Geometry: final body of the model. Coordinates: model frame, mm. Face numbers are marked on the shaded views. A direction names the side the tool comes from. Give positions to 0.01 mm unless a question says otherwise; leave off trailing zeros. Loops run counter-clockwise (first coordinate to the right, second up) from the corner with the lowest first, then second, coordinate; pieces in that order, holes last. Notation, with made-up numbers: (39, 81.25) - (47, 81.25) arc R27 cw to (47, 105.25) - close; hole circle Ø3 at (-3, 83.5). An arc over 180 degrees is marked (long way). Use one line per item in the form item = value.
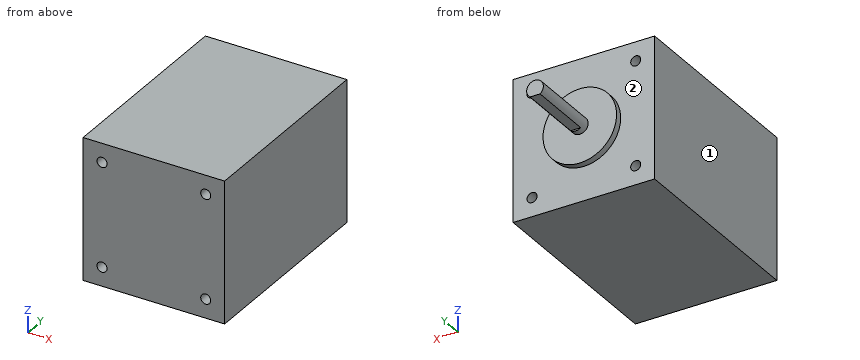
```python
from build123d import *

# Parameters (mm, degrees)
SKETCH_1_W          = 42.3
SKETCH_1_H          = 42.3
SKETCH_1_R          = 1.5
EXTRUDE_1_DEPTH     = 60
SKETCH_2_R          = 11
EXTRUDE_2_DEPTH     = 2
SKETCH_3_R          = 2.5
EXTRUDE_3_DEPTH     = 22
SKETCH_4_W          = 5
SKETCH_4_H          = 0.5
CUT_EXTRUDE_1_DEPTH = 20


with BuildPart() as part:
    # Эскиз1 → Бобышка-Вытянуть1 (new body)
    with BuildSketch(Plane(origin=(0, 0, 0), x_dir=(1, 0, 0), z_dir=(0, 1, 0))):
        with Locations((21.15, 21.15)):
            Rectangle(SKETCH_1_W, SKETCH_1_H)
        with Locations(Location((5.65, 36.65, 0), (0, 0, 270))):
            Circle(SKETCH_1_R, mode=Mode.SUBTRACT)
        with Locations(Location((36.65, 36.65, 0), (0, 0, 270))):
            Circle(SKETCH_1_R, mode=Mode.SUBTRACT)
        with Locations(Location((36.65, 5.65, 0), (0, 0, 270))):
            Circle(SKETCH_1_R, mode=Mode.SUBTRACT)
        with Locations(Location((5.65, 5.65, 0), (0, 0, 270))):
            Circle(SKETCH_1_R, mode=Mode.SUBTRACT)
    extrude(amount=EXTRUDE_1_DEPTH)

    # Эскиз2 → Бобышка-Вытянуть2 (add)
    with BuildSketch(Plane(origin=(0, 60, 0), x_dir=(1, 0, 0), z_dir=(0, 1, 0))):
        with Locations(Location((21.15, 21.15, 0), (0, 0, 90))):
            Circle(SKETCH_2_R)
    extrude(amount=EXTRUDE_2_DEPTH)

    # Эскиз3 → Бобышка-Вытянуть3 (add)
    with BuildSketch(Plane(origin=(0, 62, 0), x_dir=(1, 0, 0), z_dir=(0, 1, 0))):
        with Locations(Location((21.15, 21.15, 0), (0, 0, 270))):
            Circle(SKETCH_3_R)
    extrude(amount=EXTRUDE_3_DEPTH)

    # Эскиз4 → Вырез-Вытянуть1 (cut)
    with BuildSketch(Plane(origin=(0, 84, 0), x_dir=(1, 0, 0), z_dir=(0, 1, 0))):
        with Locations((21.15, 23.4)):
            Rectangle(SKETCH_4_W, SKETCH_4_H)
    extrude(amount=-CUT_EXTRUDE_1_DEPTH, mode=Mode.SUBTRACT)


solid = part.part
```
(1) Material intervals for L1, parallel to X at y = 23, z = -5.65; L2, parallel to X at y = 18, z = -36; L3, parallel to Z at x = 5, y = 31, sorted ascending. Write a range as from..to.
Solution:
L1 = 0..4.15, 7.15..35.15, 38.15..42.3
L2 = 0..4.3, 7..35.3, 38..42.3
L3 = -42.3..-38, -35.3..-7, -4.3..0
(2) Cut plane A-A (y = 28). Return the cut outline in (x, z).
Solution:
outline = (0, -42.3) - (42.3, -42.3) - (42.3, 0) - (0, 0) - close; hole circle Ø3 at (5.65, -36.65); hole circle Ø3 at (5.65, -5.65); hole circle Ø3 at (36.65, -36.65); hole circle Ø3 at (36.65, -5.65)
(3) Cut plane B-B (x = 5.65). Return the cut outline in (y, z), plus the area to 3 significant figures.
Solution:
outline = (0, -42.3) - (60, -42.3) - (60, -38.15) - (0, -38.15) - close; (0, -35.15) - (60, -35.15) - (60, -7.15) - (0, -7.15) - close; (0, -4.15) - (60, -4.15) - (60, 0) - (0, 0) - close
area = 2,180 mm2
(4) Cut plane C-C (z = -5.65). Return the cut outline in (x, y), plus the area to 3 significant figures.
Solution:
outline = (0, 0) - (4.15, 0) - (4.15, 60) - (0, 60) - close; (7.15, 0) - (35.15, 0) - (35.15, 60) - (7.15, 60) - close; (38.15, 0) - (42.3, 0) - (42.3, 60) - (38.15, 60) - close
area = 2,180 mm2
(5) Pin query (flat end, axial travel): P1, Ø2.5, axis at x = 5.65, z = -5.65, coming from the -Y side; P2, Ø12, axis at x = 33, z = -34, coming from the +Y side; P3, Ø2.5, axis at x = 21, y = 73.5, coming from the -Z side. Return the tip coordinate at first contact, or that it passes through.
Solution:
P1 = through
P2 = 60
P3 = -23.15
(6) Cut plane D-D (z = -21.15). Return the cut outline in (x, y).
Solution:
outline = (0, 0) - (42.3, 0) - (42.3, 60) - (32.15, 60) - (32.15, 62) - (23.65, 62) - (23.65, 84) - (18.65, 84) - (18.65, 62) - (10.15, 62) - (10.15, 60) - (0, 60) - close
(7) Access query for the marked faces 1 and 2. Directions: +Z, -Z, +X, -X, +Y, -Y. A direction counts if a zero-diameter tool reaches every point of the face in a straight line with its end or side. Return the directions, or none.
Solution:
face_1 = +Z, -Z, -X, +Y, -Y
face_2 = +Y
